```python
from build123d import *

# Parameters (mm, degrees)
BOSS_EXTRUDE1_DEPTH = 30
SKETCH2_W           = 76
SKETCH2_H           = 5
BOSS_EXTRUDE2_DEPTH = 23
SKETCH3_W           = 76
SKETCH3_H           = 5
BOSS_EXTRUDE3_DEPTH = 23
SKETCH4_W           = 8
SKETCH4_H           = 20
CUT_EXTRUDE1_DEPTH  = 5
SKETCH5_R           = 2
CUT_EXTRUDE2_DEPTH  = 20
SKETCH6_R           = 3
CUT_EXTRUDE3_DEPTH  = 5


with BuildPart() as part:
    # Sketch1 → Boss-Extrude1 (new body)
    with BuildSketch(Plane.XY):
        Polygon((0, 15), (38, 15), (38, 10), (38, -5), (4, -5), (4, -15), (0, -15), (-4, -15), (-4, -5), (-38, -5), (-38, 10), (-38, 15), align=None)
        Polygon((-2.5, -5), (2.5, -5), (2.5, -7.5), (2.5, -10), (0, -10), (-2.5, -10), (-2.5, -7.5), align=None, mode=Mode.SUBTRACT)
    extrude(amount=-BOSS_EXTRUDE1_DEPTH)

    # Sketch2 → Boss-Extrude2 (add)
    with BuildSketch(Plane.XY):
        with Locations((0, 12.5)):
            Rectangle(SKETCH2_W, SKETCH2_H)
    extrude(amount=BOSS_EXTRUDE2_DEPTH)

    # Sketch3 → Boss-Extrude3 (add)
    with BuildSketch(Plane(origin=(0, 0, -30), x_dir=(-1, 0, 0), z_dir=(0, 0, -1))):
        with Locations((0, 12.5)):
            Rectangle(SKETCH3_W, SKETCH3_H)
    extrude(amount=BOSS_EXTRUDE3_DEPTH)

    # Sketch4 → Cut-Extrude1 (cut)
    with BuildSketch(Plane(origin=(0, -15, 0), x_dir=(-1, 0, 0), z_dir=(0, -1, 0))):
        with Locations((0, 15)):
            Rectangle(SKETCH4_W, SKETCH4_H)
    extrude(amount=-CUT_EXTRUDE1_DEPTH, mode=Mode.SUBTRACT)

    # Sketch5 → Cut-Extrude2 (cut)
    with BuildSketch(Plane(origin=(0, -5, 0), x_dir=(-1, 0, 0), z_dir=(0, -1, 0))):
        with Locations(Location((33.048249635, 6.95460219, 0), (0, 0, 90))):
            Circle(SKETCH5_R)
        with Locations(Location((9.048249635, 6.95460219, 0), (0, 0, 90))):
            Circle(SKETCH5_R)
        with Locations(Location((33.048249635, 22.95460219, 0), (0, 0, 90))):
            Circle(SKETCH5_R)
        with Locations(Location((9.048249635, 22.95460219, 0), (0, 0, 90))):
            Circle(SKETCH5_R)
        with Locations(Location((-9, 7, 0), (0, 0, 90))):
            Circle(SKETCH5_R)
        with Locations(Location((-33, 7, 0), (0, 0, 90))):
            Circle(SKETCH5_R)
        with Locations(Location((-33, 23, 0), (0, 0, 90))):
            Circle(SKETCH5_R)
        with Locations(Location((-9, 23, 0), (0, 0, 90))):
            Circle(SKETCH5_R)
    extrude(amount=-CUT_EXTRUDE2_DEPTH, mode=Mode.SUBTRACT)

    # Sketch6 → Cut-Extrude3 (cut)
    with BuildSketch(Plane(origin=(0, 15, 0), x_dir=(1, 0, 0), z_dir=(0, 1, 0))):
        with Locations(Location((28, -13, 0), (0, 0, 270))):
            Circle(SKETCH6_R)
        with Locations(Location((-28, -13, 0), (0, 0, 270))):
            Circle(SKETCH6_R)
        with Locations(Location((-28, 43, 0), (0, 0, 270))):
            Circle(SKETCH6_R)
        with Locations(Location((28, 43, 0), (0, 0, 270))):
            Circle(SKETCH6_R)
    extrude(amount=-CUT_EXTRUDE3_DEPTH, mode=Mode.SUBTRACT)


solid = part.part
```
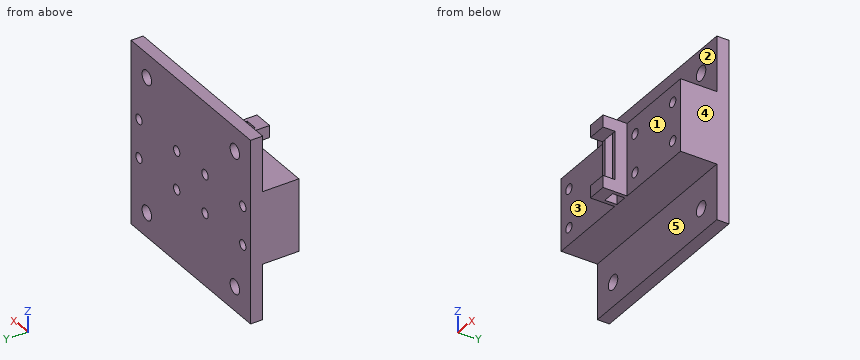
Here's how the part is built. I have some questions about the finished solid (model axes, mm). Face numbers are marked on the shaded views. A direction names the side the tool comes from. Give positions to 0.01 mm unless a question says otherwise; leave off trailing zeros. Write each loop counter-clockwise with the first axis right and the second up, starting at its lowest first coordinate (ties: lowest second). Pieces come first, ordered by that corner, then holes.
(1) Will these pins go through, and if not, where does the flat tip stop? pin 1 (3 mm diameter, centred on x = -9.05, z = -6.95, fed in from +Y); pin 2 (5 mm diameter, centred on x = 19, y = 3, fed in from -Z); pin 3 (6.5 mm diameter, centred on x = 9, z = -7, fed in from -Y); pin 4 (2.5 mm diameter, centred on y = -7, z = -8, fed in from +X).
Output values:
pin 1: passes through
pin 2: stops at z = -30
pin 3: stops at y = -5
pin 4: stops at x = 4
(2) Imagine slicing it at B-B, the plane x = 28. Write out the boundary of the cut face in (y, z), and give its area (3 significant figures).
Output values:
outline: (-5, -30) - (10, -30) - (10, -40) - (15, -40) - (15, 10) - (10, 10) - (10, 0) - (-5, 0) - close; (10, -53) - (15, -53) - (15, -46) - (10, -46) - close; (10, 16) - (15, 16) - (15, 23) - (10, 23) - close
area: 770 mm2
(3) Imagine slicing it at C-C, the plane z = 13. Write out the boundary of the cut face in (x, y).
Output values:
outline: (-38, 10) - (-31, 10) - (-31, 15) - (-38, 15) - close; (-25, 10) - (25, 10) - (25, 15) - (-25, 15) - close; (31, 10) - (38, 10) - (38, 15) - (31, 15) - close
(4) On a 3-axis mill with a long thin cutter (end or side, diameter ignored), from which of +Z, -Z, +X, -X, +Y, -Y can I reach the whole of each face in a straight line? I mean the marked faces 1, 2, 3, 4 and 5. Say none if no direction works.
Output values:
face 1: +Z, -Z, +X, -Y
face 2: +Z, +X, -X, -Y
face 3: +Z, -Z, -X, -Y
face 4: +Z, -Z, +X, +Y, -Y
face 5: -Z, +X, -X, -Y
(5) Imagine slicing it at D-D, the plane z = -23. Write out the boundary of the cut face in (x, y), and give its area (3 significant figures).
Output values:
outline: (-38, -5) - (-35.05, -5) - (-35.05, 15) - (-38, 15) - close; (-31.05, -5) - (-11.05, -5) - (-11.05, 15) - (-31.05, 15) - close; (-7.05, -5) - (-4, -5) - (-4, -10) - (-2.5, -10) - (-2.5, -5) - (2.5, -5) - (2.5, -10) - (4, -10) - (4, -5) - (7, -5) - (7, 15) - (-7.05, 15) - close; (11, -5) - (31, -5) - (31, 15) - (11, 15) - close; (35, -5) - (38, -5) - (38, 15) - (35, 15) - close
area: 1,220 mm2
(6) If I drill on L1, parallel to X at y = 11.45, z = 13; L2, parallel to Z at x = -15, y = -1.5; L3, parallel to Y at x = 27, z = -28, over which ranges is the centre line in solid material (lowest first)?
Output values:
L1: x = -38 to -31, -25 to 25, 31 to 38
L2: z = -30 to 0
L3: y = -5 to 15
(7) Imagine slicing it at A-A, the plane y = -12.5. Write out the boundary of the cut face in (x, z).
Output values:
outline: (-4, -30) - (4, -30) - (4, -25) - (-4, -25) - close; (-4, -5) - (4, -5) - (4, 0) - (-4, 0) - close
